Geometry check sheet. Reference: the model listing, model coordinates, mm. Round coordinates to 2 decimals unless told otherwise and drop trailing zeros. Write each loop counter-clockwise with the first axis right and the second up, starting at its lowest first coordinate (ties: lowest second). Pieces come first, ordered by that corner, then holes. Notation, with made-up numbers: M -15.75,38.5 L -7.75,38.5 A26 ccw -7.75,67.5 Z; hole C 12,33.25 d7. An arc over 180 degrees is marked long. Use a Markdown table: item, result.
```python
from build123d import *

# Parameters (mm, degrees)
CROQUIS1_R              = 4.5
SALIENTE_EXTRUIR1_DEPTH = 3


with BuildPart() as part:
    # Croquis1 → Saliente-Extruir1 (new body)
    with BuildSketch(Plane.XY):
        Polygon((-60, 25), (-55, 30), (55, 30), (60, 25), (60, 0), (-60, 0), align=None)
        with Locations((-50, 20)):
            Circle(CROQUIS1_R, mode=Mode.SUBTRACT)
        with Locations((50, 20)):
            Circle(CROQUIS1_R, mode=Mode.SUBTRACT)
    extrude(amount=SALIENTE_EXTRUIR1_DEPTH)


solid = part.part
```
Item 1: Mould release check, pull along Y, two halves, no side actions. Record for faces 1 (the face through (1, 0, 1)), 2 (the face through (-1, 30, 1)), 3 (the face through (54.292, 21.352, 1.479)): +Y half, -Y half, draft (parallel to the pull), parting line (faces both ways), or undercut.
Outcome:
| item | result |
|---|---|
| face 1 | -Y half |
| face 2 | +Y half |
| face 3 | undercut |
Item 2: Cross-section at C-C, the plane z = 1.25. Record the cut outline in (x, y), and give its area (3 significant figures).
Outcome:
| item | result |
|---|---|
| outline | M -60,0 L 60,0 L 60,25 L 55,30 L -55,30 L -60,25 Z; hole C -50,20 d9; hole C 50,20 d9 |
| area | 3,450 mm2 |
Item 3: Go/stop test with a flat-tipped pin: pin 1 (6 mm diameter, centred on x = -1, y = 11.5, fed in from -Z). Record where the tip stops, or that it passes through.
Outcome:
| item | result |
|---|---|
| pin 1 | stops at z = 0 |
Item 4: Cross-section at D-D, the plane x = 49. Record the cut outline in (y, z).
Outcome:
| item | result |
|---|---|
| outline | M 0,0 L 15.61,0 L 15.61,3 L 0,3 Z; M 24.39,0 L 30,0 L 30,3 L 24.39,3 Z |
Item 5: Material ranges on line 1 along X through (y, z) = (18, 2.6); line 2 along Y through (x, z) = (50, 1.4); line 3 along X through (y, z) = (20.5, 1.6), recorded low to high. Write a range as from..to.
Outcome:
| item | result |
|---|---|
| line 1 | x = -60..-54.03, -45.97..45.97, 54.03..60 |
| line 2 | y = 0..15.5, 24.5..30 |
| line 3 | x = -60..-54.47, -45.53..45.53, 54.47..60 |
Item 6: Cross-section at B-B, the plane x = -50. Record the cut outline in (y, z), and give its area (3 significant figures).
Outcome:
| item | result |
|---|---|
| outline | M 0,0 L 15.5,0 L 15.5,3 L 0,3 Z; M 24.5,0 L 30,0 L 30,3 L 24.5,3 Z |
| area | 63.0 mm2 |
Item 7: Cross-section at A-A, the plane y = 20. Record the cut outline in (x, z), and give its area (3 significant figures).
Outcome:
| item | result |
|---|---|
| outline | M -60,0 L -54.5,0 L -54.5,3 L -60,3 Z; M -45.5,0 L 45.5,0 L 45.5,3 L -45.5,3 Z; M 54.5,0 L 60,0 L 60,3 L 54.5,3 Z |
| area | 306 mm2 |
